```python
from build123d import *

# Parameters (mm, degrees)
F0_R     = 1.6
F1_DEPTH = 3
F2_R     = 1.6
F3_DEPTH = 3


with BuildPart() as f1:
    # F0 (on Front) → F1 (new body)
    with BuildSketch(Plane.XZ):
        with BuildLine():
            Line((-25, -7.5), (-4.5, -7.5))
            ThreePointArc((-4.5, -7.5), (-3.085786, -6.914214), (-2.5, -5.5))
            Line((-2.5, -5.5), (-2.5, -5))
            ThreePointArc((-2.5, -5), (-1.767767, -3.232233), (0, -2.5))
            Line((0, -2.5), (25, -2.5))
            ThreePointArc((25, -2.5), (26.767767, -1.767767), (27.5, 0))
            Line((27.5, 0), (27.5, 5))
            ThreePointArc((27.5, 5), (26.767767, 6.767767), (25, 7.5))
            Line((25, 7.5), (-25, 7.5))
            ThreePointArc((-25, 7.5), (-26.767767, 6.767767), (-27.5, 5))
            Line((-27.5, 5), (-27.5, -5))
            ThreePointArc((-27.5, -5), (-26.767767, -6.767767), (-25, -7.5))
        make_face()
        with Locations((-17.5, 0)):
            Circle(F0_R, mode=Mode.SUBTRACT)
        with Locations((12.5, 2.5)):
            Circle(F0_R, mode=Mode.SUBTRACT)
        with Locations((22.5, 2.5)):
            Circle(F0_R, mode=Mode.SUBTRACT)
    extrude(amount=F1_DEPTH)

    # F2 (on face) → F3 (join)
    with BuildSketch(Plane.XZ.offset(3)):
        with BuildLine():
            Line((-25, -7.5), (-10, -7.5))
            ThreePointArc((-10, -7.5), (-8.232233, -6.767767), (-7.5, -5))
            Line((-7.5, -5), (-7.5, 5))
            ThreePointArc((-7.5, 5), (-8.232233, 6.767767), (-10, 7.5))
            Line((-10, 7.5), (-25, 7.5))
            ThreePointArc((-25, 7.5), (-26.767767, 6.767767), (-27.5, 5))
            Line((-27.5, 5), (-27.5, -5))
            ThreePointArc((-27.5, -5), (-26.767767, -6.767767), (-25, -7.5))
        make_face()
        with Locations((-17.5, 0)):
            Circle(F2_R, mode=Mode.SUBTRACT)
    extrude(amount=F3_DEPTH)


solid = f1.part
```
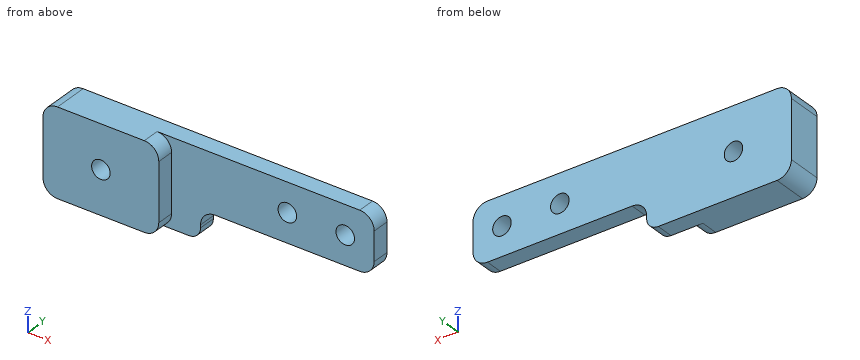
Geometry check sheet. Reference: the model listing, model coordinates, mm. Give positions to 0.01 mm unless a question says otherwise; leave off trailing zeros. Order: outer loops, then holes, each group sorted by start corner. A loop starts at its lowest first (then second) coordinate and runs counter-clockwise, first axis right, second up. Notation, with made-up numbers: (-36, -18) - (-24, -18) arc R15 cw to (-24, -12) - close; hole circle Ø3 at (85.25, -17). An arc over 180 degrees is marked (long way). Answer in a Markdown table with one row per item. Add a question column.
Q1. Cross-section at D-D, the plane y = -5.05. Enter the section's corners in (x, z), then the cut area to 3 significant figures.
Q2. Gauge pin test, flat ends, axial feed: pin 1 (4 mm diameter, centred on x = 22.5, z = 2.5, fed in from +Y); pin 2 (3 mm diameter, centred on x = -17.5, z = 0, fed in from +Y); pin 3 (2.5 mm diameter, centred on x = 10, y = -1.5, fed in from -Z); pin 4 (0.6 mm diameter, centred on y = -1.5, z = -5.5, fed in from +X). Record the tip position at first contact, or that the pin passes through.
Q3. Cross-section at C-C, the plane y = -2.05. Enter the section's corners in (x, z).
Q4. Material ranges on probe 1 along Z at (x, y) = (12.5, -1.2); probe 2 along Z at (x, y) = (-17.5, -1.2); probe 3 along Y at (x, z) = (24.5, 1.25), recorded low to high. Write a range as from..to.
Q5. Cross-section at A-A, the plane x = -17.5. Enter the section's corners in (y, z), then the cut area to 3 significant figures.
Q6. Cross-section at B-B, the plane z = 2.5. Enter the section's corners in (x, y), then the cut area to 3 significant figures.
Check values:
| question | item | result |
|---|---|---|
| 1 | outline | (-27.5, -5) arc R2.5 ccw to (-25, -7.5) - (-10, -7.5) arc R2.5 ccw to (-7.5, -5) - (-7.5, 5) arc R2.5 ccw to (-10, 7.5) - (-25, 7.5) arc R2.5 ccw to (-27.5, 5) - close; hole circle Ø3.2 at (-17.5, 0) |
| 1 | area | 287 mm^2 |
| 2 | pin 1 | stops at y = 0 |
| 2 | pin 2 | passes through |
| 2 | pin 3 | stops at z = -2.5 |
| 2 | pin 4 | stops at x = -2.5 |
| 3 | outline | (-27.5, -5) arc R2.5 ccw to (-25, -7.5) - (-4.5, -7.5) arc R2 ccw to (-2.5, -5.5) - (-2.5, -5) arc R2.5 cw to (0, -2.5) - (25, -2.5) arc R2.5 ccw to (27.5, 0) - (27.5, 5) arc R2.5 ccw to (25, 7.5) - (-25, 7.5) arc R2.5 ccw to (-27.5, 5) - close; hole circle Ø3.2 at (-17.5, 0); hole circle Ø3.2 at (12.5, 2.5); hole circle Ø3.2 at (22.5, 2.5) |
| 4 | probe 1 | z = -2.5..0.9, 4.1..7.5 |
| 4 | probe 2 | z = -7.5..-1.6, 1.6..7.5 |
| 4 | probe 3 | y = -3..0 |
| 5 | outline | (-6, -7.5) - (0, -7.5) - (0, -1.6) - (-6, -1.6) - close; (-6, 1.6) - (0, 1.6) - (0, 7.5) - (-6, 7.5) - close |
| 5 | area | 70.8 mm^2 |
| 6 | outline | (-27.5, -6) - (-7.5, -6) - (-7.5, -3) - (10.9, -3) - (10.9, 0) - (-27.5, 0) - close; (14.1, -3) - (20.9, -3) - (20.9, 0) - (14.1, 0) - close; (24.1, -3) - (27.5, -3) - (27.5, 0) - (24.1, 0) - close |
| 6 | area | 206 mm^2 |
